```python
from build123d import *

# Parameters (mm, degrees)
F1_DEPTH      = 20
F2_R          = 1
F3_DEPTH      = 10
F4_R          = 1
F5_DEPTH      = 10
F7_DEPTH      = 75
F7_DEPTH_BACK = -18
F9_DEPTH      = 12
F11_DEPTH     = 12
F12_W         = 18
F12_H         = 20
F13_DEPTH     = 7
F14_R         = 1.5
F15_DEPTH     = 25
F16_R         = 3
F18_DEPTH     = 22.5
F20_DEPTH     = 22.5
F21_R         = 1
F22_DEPTH     = 10
F23_W         = 7
F23_H         = 14
F24_DEPTH     = 7
F25_R         = 1
F26_DEPTH     = 25
F27_R         = 1
F28_DEPTH     = 10
F29_R         = 1.5
F30_R         = 1.5
F33_DEPTH     = 5
F32_R         = 1.5
F34_DEPTH     = 3


with BuildPart() as f1:
    # F0 (on Top) → F1 (new body)
    with BuildSketch(Plane.XY):
        Polygon((0, 8), (0, 0), (57, 0), (57, 8), (30, 8), (30, 50), (57, 50), (57, 65), (0, 65), (0, 50), (27, 50), (27, 8), align=None)
    extrude(amount=F1_DEPTH)

    # F2 (on face) → F3 (cut)
    with BuildSketch(Plane.YZ.offset(57)):
        with Locations((3.4, 15)):
            Circle(F2_R)
        with Locations((3.4, 5)):
            Circle(F2_R)
        with Locations((53.9, 15)):
            Circle(F2_R)
        with Locations((53.9, 5)):
            Circle(F2_R)
    extrude(amount=-F3_DEPTH, mode=Mode.SUBTRACT)

    # F4 (on face) → F5 (cut)
    with BuildSketch(Plane(origin=(0, 0, 0), x_dir=(0, -1, 0), z_dir=(-1, 0, 0))):
        with Locations((-53.9, 15)):
            Circle(F4_R)
        with Locations((-53.9, 5)):
            Circle(F4_R)
        with Locations((-3.4, 15)):
            Circle(F4_R)
        with Locations((-3.4, 5)):
            Circle(F4_R)
    extrude(amount=-F5_DEPTH, mode=Mode.SUBTRACT)

    # F6 (on face) → F7 (join, two sides)
    with BuildSketch(Plane.YZ.offset(57)) as f7_sk:
        Polygon((65, 20), (65, 5), (95, 20), align=None)
    extrude(amount=-F7_DEPTH)
    extrude(f7_sk.sketch, amount=-F7_DEPTH_BACK)

    # F8 (on face) → F9 (cut)
    with BuildSketch(Plane.XZ):
        Polygon((27, 0), (27, 13), (22.5, 13), (22.5, 7), (22.5, 0), align=None)
        Polygon((30, 13), (30, 0), (34.5, 0), (34.5, 7), (34.5, 13), align=None)
    extrude(amount=-F9_DEPTH, mode=Mode.SUBTRACT)

    # F10 (on face) → F11 (cut)
    with BuildSketch(Plane(origin=(0, 0, 0), x_dir=(1, 0, 0), z_dir=(0, 0, -1))):
        Polygon((27, -105), (27, -65), (0, -65), (-23, -65), (-23, -105), align=None)
        Polygon((57, -65), (30, -65), (30, -105), (80, -105), (80, -65), align=None)
    extrude(amount=-F11_DEPTH, mode=Mode.SUBTRACT)

    # F12 (on face) → F13 (join)
    with BuildSketch(Plane(origin=(0, 65, 0), x_dir=(-1, 0, 0), z_dir=(0, 1, 0))):
        with Locations((-66, 10)):
            Rectangle(F12_W, F12_H)
        with Locations((9, 10)):
            Rectangle(F12_W, F12_H)
    extrude(amount=-F13_DEPTH)

    # F14 (on face) → F15 (cut)
    with BuildSketch(Plane(origin=(0, 65, 0), x_dir=(-1, 0, 0), z_dir=(0, 1, 0))):
        with Locations((-71.5, 5.7)):
            Circle(F14_R)
        with Locations((-34.5, 5.7)):
            Circle(F14_R)
        with Locations((-22.5, 5.7)):
            Circle(F14_R)
        with Locations((14.5, 5.7)):
            Circle(F14_R)
    extrude(amount=-F15_DEPTH, mode=Mode.SUBTRACT)

    # F16
    f16_edges = [f1.edges().sort_by_distance(p)[0] for p in [
        (75, 61.5, 0),
        (-18, 61.5, 0),
    ]]
    fillet(f16_edges, radius=F16_R)

    # F17 (on face) → F18 (join, through all)
    with BuildSketch(Plane.YZ.offset(57)):
        Polygon((-3, 8), (-3, 0), (0, 0), (0, 20), align=None)
    extrude(amount=-F18_DEPTH)

    # F19 (on face) → F20 (join, through all)
    with BuildSketch(Plane(origin=(0, 0, 0), x_dir=(0, -1, 0), z_dir=(-1, 0, 0))):
        Polygon((0, 0), (3, 0), (3, 8), (0, 20), align=None)
    extrude(amount=-F20_DEPTH)

    # F21 (on face) → F22 (cut)
    with BuildSketch(Plane(origin=(0, 0, 0), x_dir=(1, 0, 0), z_dir=(0, 0, -1))):
        with Locations((5.5, -57)):
            Circle(F21_R)
        with Locations((5.5, 3)):
            Circle(F21_R)
        with Locations((51.5, 3)):
            Circle(F21_R)
        with Locations((51.5, -57)):
            Circle(F21_R)
    extrude(amount=-F22_DEPTH, mode=Mode.SUBTRACT)

    # F23 (on face) → F24 (cut)
    with BuildSketch(Plane.XY.offset(20)):
        with Locations((-6.5, 65)):
            Rectangle(F23_W, F23_H)
        with Locations((63.5, 65)):
            Rectangle(F23_W, F23_H)
    extrude(amount=-F24_DEPTH, mode=Mode.SUBTRACT)

    # F25 (on face) → F26 (cut)
    with BuildSketch(Plane.XZ.offset(3)):
        with Locations((17.5, 4)):
            Circle(F25_R)
        with Locations((39.5, 4)):
            Circle(F25_R)
    extrude(amount=-F26_DEPTH, mode=Mode.SUBTRACT)

    # F27 (on face) → F28 (cut)
    with BuildSketch(Plane.XY.offset(13)):
        with Locations((-7.5, 60.5)):
            Circle(F27_R)
        with Locations((62.5, 60.5)):
            Circle(F27_R)
    extrude(amount=-F28_DEPTH, mode=Mode.SUBTRACT)

    # F29 (on face) + F30 (on face) → F33 (cut)
    with BuildSketch(Plane.XZ.offset(-50)):
        Polygon((34.5, 2.524574), (37.25, 4.112287), (37.25, 7.287713), (34.5, 8.875426), (31.75, 7.287713), (31.75, 4.112287), align=None)
        with Locations((34.5, 5.7)):
            Circle(F29_R, mode=Mode.SUBTRACT)
    with BuildSketch(Plane.XZ.offset(-50)):
        Polygon((19.75, 7.287713), (19.75, 4.112287), (22.5, 2.524574), (25.25, 4.112287), (25.25, 7.287713), (22.5, 8.875426), align=None)
        with Locations((22.5, 5.7)):
            Circle(F30_R, mode=Mode.SUBTRACT)
    extrude(amount=-F33_DEPTH, mode=Mode.SUBTRACT)

    # F31 (on face) + F32 (on face) → F34 (cut)
    with BuildSketch(Plane.XZ.offset(-58)):
        Polygon((71.5, 8.875426), (68.75, 7.287713), (68.75, 4.112287), (71.5, 2.524574), (74.25, 4.112287), (74.25, 7.287713), align=None)
    with BuildSketch(Plane.XZ.offset(-58)):
        Polygon((-11.75, 4.112287), (-11.75, 7.287713), (-14.5, 8.875426), (-17.25, 7.287713), (-17.25, 4.112287), (-14.5, 2.524574), align=None)
        with Locations((-14.5, 5.7)):
            Circle(F32_R, mode=Mode.SUBTRACT)
    extrude(amount=-F34_DEPTH, mode=Mode.SUBTRACT)


solid = f1.part
```
Work out the finished part from the listing and answer in its coordinate system (mm). A direction names the side the tool comes from. Give positions to 0.01 mm unless a question says otherwise; leave off trailing zeros. Write each loop counter-clockwise with the first axis right and the second up, starting at its lowest first coordinate (ties: lowest second). Pieces come first, ordered by that corner, then holes. Notation, with made-up numbers: (56, -25.75) -> (86, -25.75) arc R7 cw to (86, -16.75) -> close; hole circle Ø2 at (60.25, 7). An arc over 180 degrees is marked (long way). Write each question's results on one line, items separated by ' | '.
1. Each of these flat-tipped pins is pushed along its axis until it touches: pin 1 Ø1.8 at (y, z) = (53.9, 15) entering from -X; pin 2 Ø3 at (y, z) = (7, 17.5) entering from +X; pin 3 Ø1.6 at (y, z) = (3.5, 14.5) entering from -X; pin 4 Ø1.5 at (x, y) = (-1, 48.5) entering from -Z. Where does it stop, or does it pass through?
Data:
pin 1: x = 10 | pin 2: x = 57 | pin 3: x = 0 | pin 4: through
2. Straight lines are drawn through the part: L1, parallel to Z at x = 53.5, y = 3.4; L2, parallel to X at y = 57, z = 2.75; L3, parallel to Y at x = 53.5, z = 3. For each, find the intervals that lie inside material, in ascending order.
Data:
L1: 0 to 4, 6 to 14, 16 to 20 | L2: 0 to 4.5, 6.5 to 50.5, 52.5 to 57 | L3: -3 to 8, 50 to 65
3. A tool of negligible diameter and unlimited length cuts with its end or side. For faces 5 (the flat face through (34, 55, 4)), 6 (the flat face through (-3, 65, 17)), 7 (the flat face through (-13.106, 59.479, 8.07)), from which of +Z, -Z, +X, -X, +Y, -Y can it reach the whole face along a straight path? Write none if from no direction.
Data:
face 5: none | face 6: +Z, -Y | face 7: -Y
4. Find section A-A on y = 32. Determine the outline of the cut face in (x, z).
Data:
outline: (27, 0) -> (30, 0) -> (30, 20) -> (27, 20) -> close
5. Determine the mould class of faces 1 (the flat face through (0, 3, 10)), 2 (the cylindrical face through (-17.1, 61.45, 0.86)), 3 (the flat face through (-11.75, 59, 6)), 4 (the flat face through (25.25, 52, 6)) for opening direction Z: +Z half, -Z half, draft (parallel to the pull), parting line (faces both ways), or undercut.
Data:
face 1: draft | face 2: -Z half | face 3: undercut | face 4: undercut
